Source: three-view drawing plus pictorial views. Frame: mm from the lowest corner of the part. Give positions to 0.01 mm unless a question says otherwise; leave off trailing zeros. Order: outer loops, then holes, each group sorted by start corner. A loop starts at its lowest first (then second) coordinate and runs counter-clockwise, first axis right, second up.
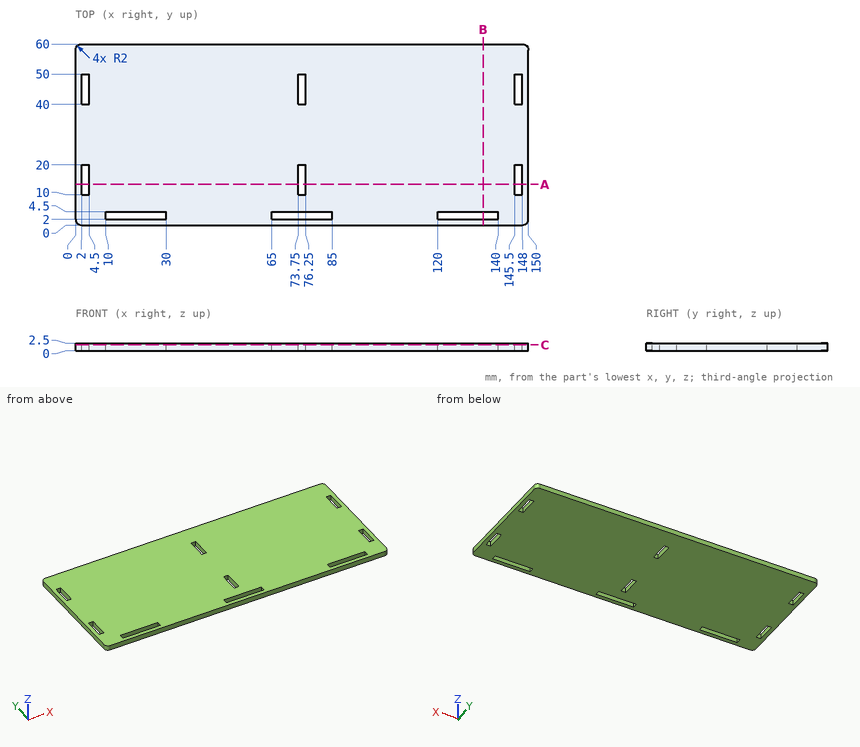
1) Section query B-B on x = 135. Output: boundary loops of the cut face in (y, z).
Checks:
outline: (0, 0) - (2, 0) - (2, 2.5) - (0, 2.5) - close; (4.5, 0) - (60, 0) - (60, 2.5) - (4.5, 2.5) - close
2) Section query C-C on z = 1.95. State how many separate pieces and enclosed holes the cut face has, and give its area (3 significant figures).
Checks:
separate pieces: 1
enclosed holes: 9
area: 8,700 mm2
3) Ray query, L1, parallel to X at y = 44, z = 1.6; L2, parallel to Y at x = 137.5, z = 0.9. Return the intervals inside material, ascending.
Checks:
L1: x = 0 to 2, 4.5 to 73.75, 76.25 to 145.5, 148 to 150
L2: y = 0 to 2, 4.5 to 60
4) Section query A-A on y = 13.5. Output: boundary loops of the cut face in (x, z).
Checks:
outline: (0, 0) - (2, 0) - (2, 2.5) - (0, 2.5) - close; (4.5, 0) - (73.75, 0) - (73.75, 2.5) - (4.5, 2.5) - close; (76.25, 0) - (145.5, 0) - (145.5, 2.5) - (76.25, 2.5) - close; (148, 0) - (150, 0) - (150, 2.5) - (148, 2.5) - close
